Part print with two shaded views. Sizes in mm from the minimum x, y, z corner. A direction names the side the tool comes from. Round coordinates to 2 decimals unless told otherwise and drop trailing zeros. Loops run counter-clockwise (first coordinate to the right, second up) from the corner with the lowest first, then second, coordinate; pieces in that order, holes last. Notation, with made-up numbers: (-21, 65.25) - (-7, 65.25) arc R25 ccw to (-7, 102.25) - close; hole circle Ø9 at (29, 47.5). An arc over 180 degrees is marked (long way). Put each result on its own line as item: value. Start each with the question number.
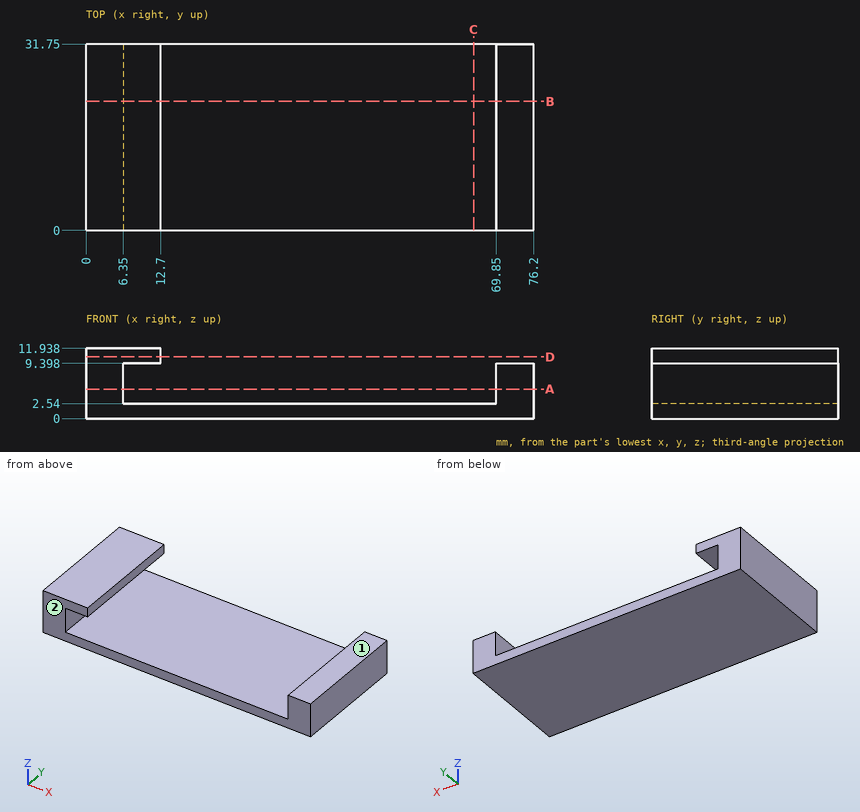
1) Slice it at D-D, the plane z = 10.5. Write the cut outline in (x, y), and give its area (3 significant figures).
2) Slice it at C-C, the plane x = 66. Write the cut outline in (y, z).
3) Slice it at A-A, the plane z = 5. Write the cut outline in (x, y), and give its area (3 significant figures).
4) Drill centre lines: line 1 (X direction, y = 13, z = 5); line 2 (X direction, y = 3, z = 9.5); line 3 (Z direction, x = 42.5, y = 27.5). Where is each one in solid material? Low to high. Write a range as [from, to].
5) Slice it at B-B, the plane y = 22. Write the cut outline in (x, z), and give its area (3 significant figures).
6) Which spindle directions (+Z, -Z, +X, -X, +Y, -Y) get a long thin tool onto all of the face, cutting with end or side? Do the marked faces 1 and 2. Say none if no direction does.
7) Drop flat-ended pins along their axis: pin 1 Ø0.8 at (y, z) = (9, 10.5) entering from +X; pin 2 Ø5 at (x, y) = (71.5, 19) entering from +Z; pin 3 Ø16 at (x, y) = (48.5, 15) entering from +Z. Give the stop position or say it passes through.
Taken from the geometry:
1. outline: (0, 0) - (12.7, 0) - (12.7, 31.75) - (0, 31.75) - close
1. area: 403 mm2
2. outline: (0, 0) - (31.75, 0) - (31.75, 2.54) - (0, 2.54) - close
3. outline: (0, 0) - (6.35, 0) - (6.35, 31.75) - (0, 31.75) - close; (69.85, 0) - (76.2, 0) - (76.2, 31.75) - (69.85, 31.75) - close
3. area: 403 mm2
4. line 1: x = [0, 6.35], [69.85, 76.2]
4. line 2: x = [0, 12.7]
4. line 3: z = [0, 2.54]
5. outline: (0, 0) - (76.2, 0) - (76.2, 9.4) - (69.85, 9.4) - (69.85, 2.54) - (6.35, 2.54) - (6.35, 9.4) - (12.7, 9.4) - (12.7, 11.94) - (0, 11.94) - close
5. area: 313 mm2
6. face 1: +Z, +X, +Y, -Y
6. face 2: +Z, -Z, +X, -X, -Y
7. pin 1: stops at x = 12.7
7. pin 2: stops at z = 9.4
7. pin 3: stops at z = 2.54
